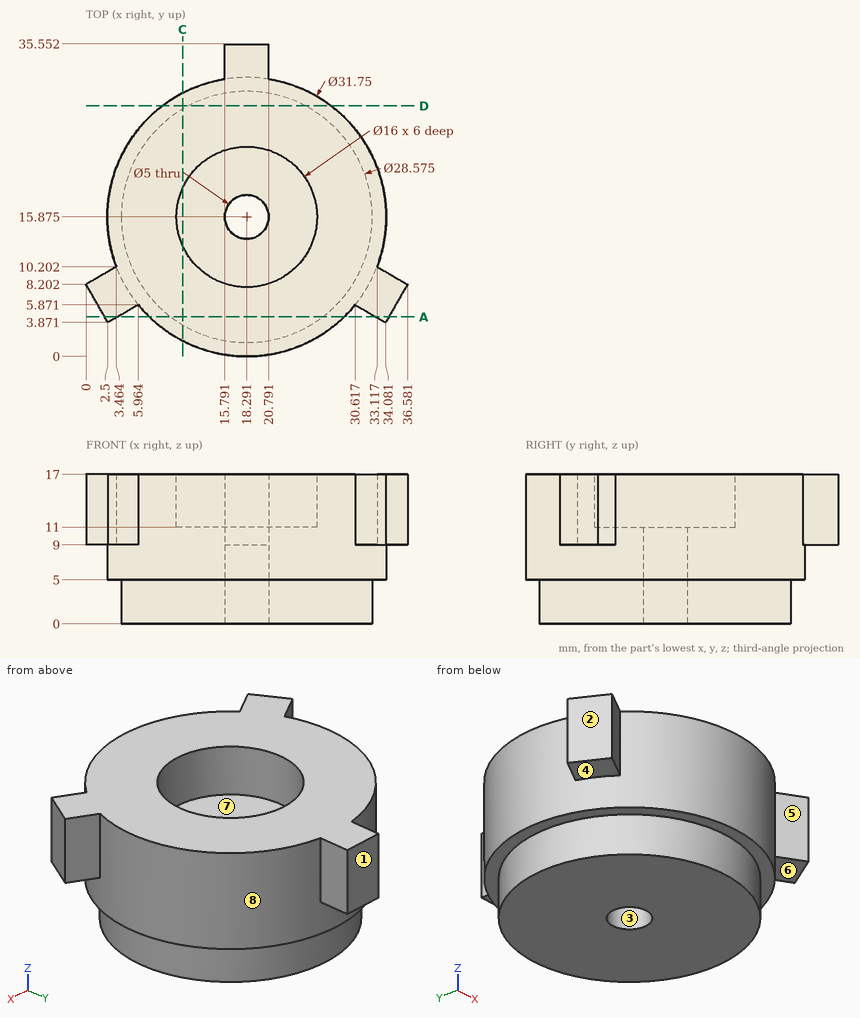
Geometry check sheet. Reference: drawing and pictorial views, mm from the part's lowest x, y, z. A direction names the side the tool comes from. Round coordinates to 2 decimals unless told otherwise and drop trailing zeros. Loops run counter-clockwise (first coordinate to the right, second up) from the corner with the lowest first, then second, coordinate; pieces in that order, holes last. Notation, with made-up numbers: (61.25, 6.5) - (72.25, 6.5) arc R27 cw to (72.25, 37.5) - close; hole circle Ø11 at (28.5, -6). An arc over 180 degrees is marked (long way). One line per question, with ' | ' between items. Start each with the question number.
1. Draft check along X on the marked faces 1, 2 and 3. Enter one of: released by +X, released by -X, zero draft, split by the parting line, or undercut.
2. Depth check by flat-ended pin: pin 1 (1 mm diameter, centred on y = 3.5, z = 7.5, fed in from -X) (1 decimal); pin 2 (4.5 mm diameter, centred on y = 32.5, z = 13, fed in from -X) (1 decimal); pin 3 (2 mm diameter, centred on y = 12.5, z = 7, fed in from +X); pin 4 (1 mm diameter, centred on x = 4.5, y = 26, fed in from +Z). Enter the tip coordinate at first touch or a pass-through.
3. Scan lines: line 1 (Y direction, x = 18.5, z = 2); line 2 (Z direction, x = 15.5, y = 30); line 3 (X direction, y = 16, z = 15.75) (1 decimal). Record each from-to range of solid material in increasing order. Write a range as [from, to].
4. Cross-section at D-D on y = 28.5. Record the cut outline in (x, z) (1 decimal).
5. Cross-section at A-A on y = 4.5. Record the cut outline in (x, z) (1 decimal).
6. Tool access check on the marked faces 4, 5, 6, 7 and 8. Record the directions out of +Z, -Z, +X, -X, +Y, -Y that give a thin tool (end or side, any length) a straight path to the whole face; none if there is none.
7. Cross-section at C-C on x = 11. Record the cut outline in (y, z), then the cut area to 3 significant figures.
Taken from the geometry:
1) face 1: zero draft | face 2: released by -X | face 3: undercut
2) pin 1: x = 7.8 | pin 2: x = 11.6 | pin 3: x = 33.99 | pin 4: through
3) line 1: [1.59, 13.38], [18.37, 30.16] | line 2: [5, 17] | line 3: [2.4, 10.3], [26.3, 34.2]
4) outline: (8.7, 5) - (11.6, 5) - (11.6, 0) - (25, 0) - (25, 5) - (27.9, 5) - (27.9, 17) - (8.7, 17) - close
5) outline: (2.1, 9) - (3.6, 9) - (3.6, 17) - (2.1, 17) - close; (7.2, 5) - (9.6, 5) - (9.6, 0) - (26.9, 0) - (26.9, 5) - (29.4, 5) - (29.4, 17) - (7.2, 17) - close; (33, 9) - (34.4, 9) - (34.4, 17) - (33, 17) - close
6) face 4: -Z, -X, -Y | face 5: +Z, -Z, -Y | face 6: -Z, +X, -Y | face 7: +Z | face 8: -Z
7) outline: (1.77, 5) - (3.59, 5) - (3.59, 0) - (28.16, 0) - (28.16, 5) - (29.98, 5) - (29.98, 17) - (19.17, 17) - (19.17, 11) - (12.58, 11) - (12.58, 17) - (1.77, 17) - close | area: 422 mm²
